Check sheet for the drawn part. Datum: minimum x, y, z corner. Units: mm. A direction names the side the tool comes from. Coordinates: 2 decimals unless noted, no trailing zeros. Loops run counter-clockwise (first coordinate to the right, second up) from the corner with the lowest first, then second, coordinate; pieces in that order, holes last. Notation, with made-up numbers: (-31, -10.75) - (-8, -10.75) arc R14 cw to (-8, 10.25) - close; hole circle Ø2 at (-22.75, -28). An arc over 180 degrees is marked (long way). Write item = value, one per line. Start each with the question number.
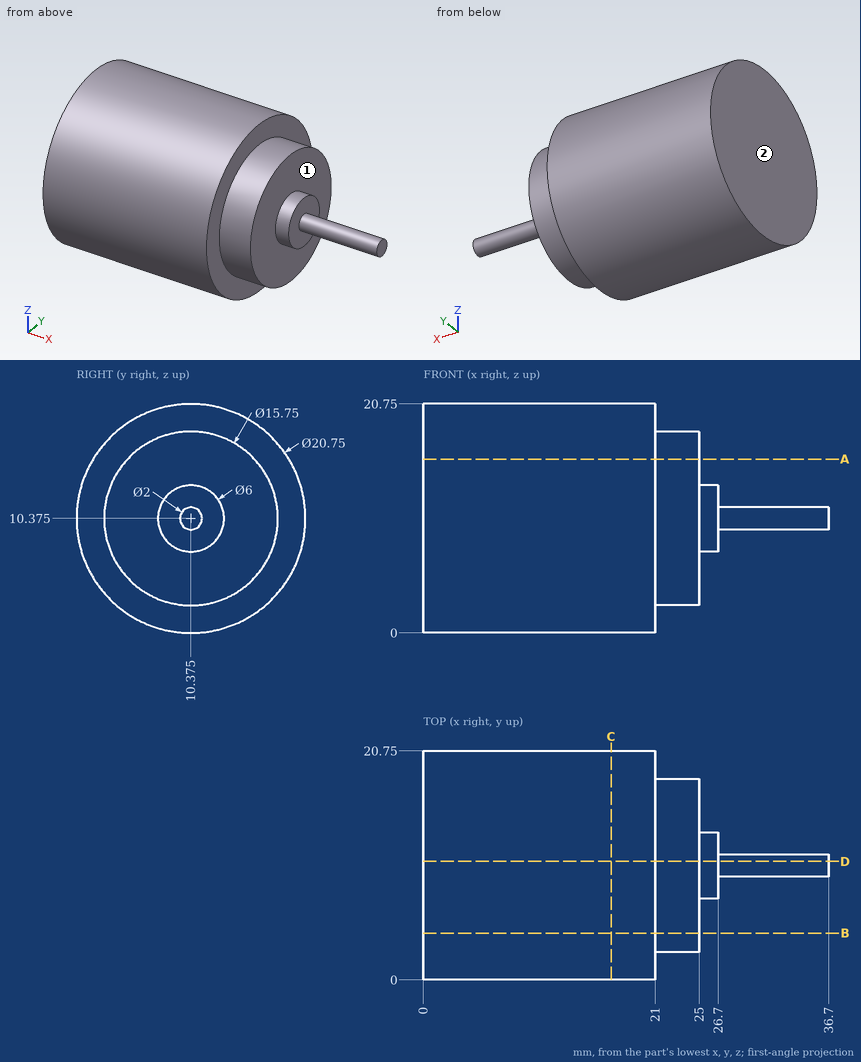
(1) Sectioned sample at D-D on y = 10.75. Enter the section's corners in (x, z), plus the area to 3 significant figures.
(2) Tool access check on the marked faces 1 and 2. Record the directions out of +Z, -Z, +X, -X, +Y, -Y that give a thin tool (end or side, any length) a straight path to the whole face; none if there is none.
(3) Depth check by flat-ended pin: pin 1 (2 mm diameter, centred on x = 16, y = 8.5, fed in from -Z); pin 2 (1 mm diameter, centred on x = 11, y = 18, fed in from -Z); pin 3 (4 mm diameter, centred on y = 14.5, z = 12, fed in from +X); pin 4 (5 mm diameter, centred on y = 11.5, z = 11, fed in from +X). Enter the tip coordinate at first touch or a pass-through.
(4) Scan lines: line 1 (X direction, y = 13.5, z = 3.5); line 2 (X direction, y = 12.25, z = 8.5); line 3 (Y direction, x = 6.5, z = 4). Record each from-to range of solid material in increasing order.
(5) Sectioned sample at C-C on x = 17. Enter the section's corners in (y, z) (3 decimals).
(6) Sectioned sample at B-B on y = 4.25. Enter the section's corners in (x, z).
(7) Sectioned sample at A-A on z = 15.75. Enter the section's corners in (x, y).
Working result:
q1.outline = (0, 0.01) - (21, 0.01) - (21, 2.51) - (25, 2.51) - (25, 7.4) - (26.7, 7.4) - (26.7, 9.45) - (36.7, 9.45) - (36.7, 11.3) - (26.7, 11.3) - (26.7, 13.35) - (25, 13.35) - (25, 18.24) - (21, 18.24) - (21, 20.74) - (0, 20.74) - close
q1.area = 527 mm2
q2.face_1 = +X
q2.face_2 = +Z, -Z, -X, +Y, -Y
q3.pin_1 = 0.04
q3.pin_2 = 2.83
q3.pin_3 = 26.7
q3.pin_4 = 36.7
q4.line_1 = 0 to 25
q4.line_2 = 0 to 26.7
q4.line_3 = 2.19 to 18.56
q5.outline = circle Ø20.75 at (10.375, 10.375)
q6.outline = (0, 2) - (21, 2) - (21, 5.43) - (25, 5.43) - (25, 15.32) - (21, 15.32) - (21, 18.75) - (0, 18.75) - close
q7.outline = (0, 1.5) - (21, 1.5) - (21, 4.62) - (25, 4.62) - (25, 16.13) - (21, 16.13) - (21, 19.25) - (0, 19.25) - close
